from build123d import *

# Parameters (mm, degrees)
SKETCH2_R            = 6.35
SKETCH2_R_2          = 4.7625
SKETCH2_R_3          = 3.5000057
BOSS_EXTRUDE1_DEPTH  = 7.62
SKETCH3_R            = 4.7625
SKETCH3_R_2          = 3.5000057
CUT_EXTRUDE1_DEPTH   = 4.445
M4_CLEARANCE_HOLE1_D = 4.8
CUT_EXTRUDE2_DEPTH   = 4.445
CIRPATTERN1_COUNT    = 4


with BuildPart() as part:
    # Sketch2 → Boss-Extrude1 (new body)
    # profile 1 of 3: a face of its own
    with BuildSketch(Plane.XY):
        with Locations(Location((0, 0, 0), (0, 0, 180))):
            Circle(SKETCH2_R)
        Circle(SKETCH2_R_2, mode=Mode.SUBTRACT)
    # profile 2 of 3: a face of its own
    with BuildSketch(Plane.XY):
        Circle(SKETCH2_R_2)
        Circle(SKETCH2_R_3, mode=Mode.SUBTRACT)
    # profile 3 of 3: a face of its own
    with BuildSketch(Plane.XY):
        Circle(SKETCH2_R_3)
    extrude(amount=BOSS_EXTRUDE1_DEPTH)

    # Sketch3 → Cut-Extrude1 (cut)
    # profile 1 of 2: a face of its own
    with BuildSketch(Plane.XY.offset(7.62)):
        Circle(SKETCH3_R)
        Circle(SKETCH3_R_2, mode=Mode.SUBTRACT)
    # profile 2 of 2: a face of its own
    with BuildSketch(Plane.XY.offset(7.62)):
        Circle(SKETCH3_R_2)
    extrude(amount=-CUT_EXTRUDE1_DEPTH, mode=Mode.SUBTRACT)

    # M4 Clearance Hole1 (through all)
    with Locations(Plane.XY.offset(3.175)):
        with Locations((0, 0)):
            Hole(M4_CLEARANCE_HOLE1_D / 2)

    # Sketch6 → Cut-Extrude2 (cut)
    with BuildSketch(Plane.XY.offset(7.62)):
        with BuildLine():
            ThreePointArc((1.5875, 6.148361062), (0, 6.35), (-1.5875, 6.148361062))
            Line((-1.5875, 6.148361062), (-1.5875, 4.490128061))
            ThreePointArc((-1.5875, 4.490128061), (0, 4.7625), (1.5875, 4.490128061))
            Line((1.5875, 4.490128061), (1.5875, 6.148361062))
        make_face()
    cut_extrude2 = extrude(amount=-CUT_EXTRUDE2_DEPTH, mode=Mode.SUBTRACT)

    # CirPattern1: Cut-Extrude2 ×4 about axis
    cirpattern1_axis = Axis((0, 0, 0), (0, 0, 1))
    for i in range(1, CIRPATTERN1_COUNT):
        add(cut_extrude2.rotate(cirpattern1_axis, i * 360 / CIRPATTERN1_COUNT), mode=Mode.SUBTRACT)


solid = part.part
Here's how the part is built. I have some questions about the finished solid (model axes, mm). A direction names the side the tool comes from. Coordinates: 2 decimals unless noted, no trailing zeros. Order: outer loops, then holes, each group sorted by start corner. A loop starts at its lowest first (then second) coordinate and runs counter-clockwise, first axis right, second up. Notation, with made-up numbers: M 52.25,23.25 L 91.25,23.25 A24 cw 91.25,33.25 Z; hole C -10,-35.5 d11. An arc over 180 degrees is marked long. Answer as CSV lines item,"result".
Item 1: For pin 1 (1.3 mm diameter, centred on x = 5.5, z = 5.5, fed in from -Y); pin 2 (0.5 mm diameter, centred on x = -5.5, z = 5.5, fed in from -Y); pin 3 (1.3 mm diameter, centred on y = -5, z = 5, fed in from -X), each with a flat end and sliding along its axis, tell me the tip position at first contact or that it passes through.
Results found:
pin 1,"y = -4.1"
pin 2,"y = -3.57"
pin 3,"x = -4.63"
Item 2: Imagine slicing it at A-A on x = 0. Write out the boundary of the cut face in (y, z) (3 decimals), plus the area to 3 significant figures.
Results found:
outline,"M -6.35,0 L -2.4,0 L -2.4,3.175 L -6.35,3.175 Z; M 2.4,0 L 6.35,0 L 6.35,3.175 L 2.4,3.175 Z"
area,"25.1 mm2"
Item 3: Imagine slicing it at B-B on z = 5.75. Give the number of separate pieces and of enclosed holes in the cut face, plus the area to 3 significant figures.
Results found:
separate pieces,"4"
enclosed holes,"0"
area,"35.0 mm2"
Item 4: We'd pull the mould along X, two halves only. Please class faces 5 (the face through (-1.588, 5, 5)), 6 (the face through (-5, -1.587, 5)), 7 (the face through (3.389, 3.347, 5.429)), 8 (the face through (-6.057, -1.907, 3.757)): +X half, -X half, draft (parallel to the pull), parting line (faces both ways), or undercut.
Results found:
face 5,"undercut"
face 6,"draft"
face 7,"undercut"
face 8,"parting line"
Item 5: On a 3-axis mill with a long thin cutter (end or side, diameter ignored), from which of +Z, -Z, +X, -X, +Y, -Y can I reach the whole of each face in a straight line? I mean faces 1 (the face through (0, -3, 3.175)), 2 (the face through (1.587, -5, 5)), 3 (the face through (4, 4, 7.62)), 4 (the face through (5, 1.587, 5)). Say none if no direction works.
Results found:
face 1,"+Z"
face 2,"+Z, +Y, -Y"
face 3,"+Z, +X, -X, +Y, -Y"
face 4,"+Z, +X, -X"
Item 6: Imagine slicing it at D-D on x = -3.5. Write out the boundary of the cut face in (y, z) (3 decimals).
Results found:
outline,"M -5.298,0 L 5.298,0 L 5.298,7.62 L 3.23,7.62 L 3.23,3.175 L -3.23,3.175 L -3.23,7.62 L -5.298,7.62 Z"
Item 7: If I drill on line 1 (Y direction, x = 0, z = 0.75); line 2 (Y direction, x = 3.5, z = 5.75); line 3 (Z direction, x = 1, y = 5) (3 decimals), over which ranges is the centre line in solid material (lowest first)?
Results found:
line 1,"-6.35 to -2.4, 2.4 to 6.35"
line 2,"-5.3 to -3.23, 3.23 to 5.3"
line 3,"0 to 3.175"
